Part model, mm, in its own coordinate system. A direction names the side the tool comes from. Give positions to 0.01 mm unless a question says otherwise; leave off trailing zeros. Write each loop counter-clockwise with the first axis right and the second up, starting at its lowest first coordinate (ties: lowest second). Pieces come first, ordered by that corner, then holes.
```python
from build123d import *

# Parameters (mm, degrees)
SKETCH1_W             = 3
SKETCH1_H             = 35
BOSS_EXTRUDE1_DEPTH   = 22
BOSS_EXTRUDE1_2_DEPTH = 22
SKETCH2_R             = 1.3
CUT_EXTRUDE1_DEPTH    = 45.891535951
SKETCH4_W             = 3
SKETCH4_H             = 35
BOSS_EXTRUDE3_DEPTH   = 8
BOSS_EXTRUDE4_DEPTH   = 3
SKETCH7_R             = 13.5
BOSS_EXTRUDE5_DEPTH   = 5
SKETCH8_R             = 11.75
CUT_EXTRUDE2_DEPTH    = 3
SKETCH9_R             = 2.5
CUT_EXTRUDE3_DEPTH    = 1.5
CUT_EXTRUDE4_START    = -1.5
SKETCH10_R            = 2.5
CUT_EXTRUDE4_DEPTH    = 1.5
SKETCH11_W            = 35
SKETCH11_H            = 3
BOSS_EXTRUDE6_DEPTH   = 17.5
SKETCH13_W            = 35
SKETCH13_H            = 3
BOSS_EXTRUDE7_DEPTH   = 40
SKETCH14_W            = 42
SKETCH14_H            = 27
BOSS_EXTRUDE8_DEPTH   = 3
SKETCH15_R            = 1.7
CUT_EXTRUDE5_DEPTH    = 40
FILLET1_R             = 10
FILLET2_R             = 5
FILLET3_R             = 3


with BuildPart() as part:
    # Sketch1 → Boss-Extrude1 (new body)
    with BuildSketch(Plane(origin=(0, 0, 0), x_dir=(1, 0, 0), z_dir=(0, 1, 0))):
        with Locations((-16, 0)):
            Rectangle(SKETCH1_W, SKETCH1_H)
    extrude(amount=BOSS_EXTRUDE1_DEPTH)


with BuildPart() as body_2:
    # Sketch1 → Boss-Extrude1 2 (new body)
    with BuildSketch(Plane(origin=(0, 0, 0), x_dir=(1, 0, 0), z_dir=(0, 1, 0))):
        with Locations((16, 0)):
            Rectangle(SKETCH1_W, SKETCH1_H)
    extrude(amount=BOSS_EXTRUDE1_2_DEPTH)


with BuildPart() as cut_extrude1_tool:
    # Sketch2 → Cut-Extrude1 (new, through all)
    with BuildSketch(Plane.ZY.offset(17.5)):
        with Locations((-12.5, 17)):
            Circle(SKETCH2_R)
        with Locations((11.5, 17)):
            Circle(SKETCH2_R)
        with Locations((11.5, 5)):
            Circle(SKETCH2_R)
        with Locations((-12.5, 5)):
            Circle(SKETCH2_R)
    extrude(amount=-CUT_EXTRUDE1_DEPTH)


with BuildPart() as part_1:
    add(part.part)

    # Cut-Extrude1: cut by cut_extrude1_tool
    add(cut_extrude1_tool.part, mode=Mode.SUBTRACT)



with BuildPart() as body_2_1:
    add(body_2.part)

    # Cut-Extrude1: cut by cut_extrude1_tool
    add(cut_extrude1_tool.part, mode=Mode.SUBTRACT)


with BuildPart() as part_2:
    add(part_1.part)

    add(body_2_1.part)  # Boss-Extrude3 merges body 2
    # Sketch4 → Boss-Extrude3 (add)
    with BuildSketch(Plane.XZ):
        with Locations((-16, 0)):
            Rectangle(SKETCH4_W, SKETCH4_H)
        with Locations((16, 0)):
            Rectangle(SKETCH4_W, SKETCH4_H)
    extrude(amount=BOSS_EXTRUDE3_DEPTH)

    # Sketch5 → Boss-Extrude4 (add)
    with BuildSketch(Plane.XZ.offset(8)):
        Polygon((-17.5, 17.5), (17.5, 17.5), (17.5, -17.5), (7.5, -17.5), (7.5, 0), (-7.5, 0), (-7.5, -17.5), (-17.5, -17.5), align=None)
    extrude(amount=BOSS_EXTRUDE4_DEPTH)

    # Sketch7 → Boss-Extrude5 (add)
    with BuildSketch(Plane.XZ.offset(11)):
        with Locations(Location((0, 16.5, 0), (0, 0, 175.751977333))):
            Circle(SKETCH7_R)
    extrude(amount=BOSS_EXTRUDE5_DEPTH)

    # Sketch8 → Cut-Extrude2 (cut)
    with BuildSketch(Plane(origin=(0, -16, 0), x_dir=(-1, 0, 0), z_dir=(0, -1, 0))):
        with Locations(Location((0, -16.5, 0), (0, 0, 90))):
            Circle(SKETCH8_R)
    extrude(amount=-CUT_EXTRUDE2_DEPTH, mode=Mode.SUBTRACT)

    # Sketch9 → Cut-Extrude3 (cut)
    with BuildSketch(Plane.ZY.offset(17.5)):
        with Locations((-12.5, 17)):
            Circle(SKETCH9_R)
        with Locations((11.5, 17)):
            Circle(SKETCH9_R)
        with Locations((11.5, 5)):
            Circle(SKETCH9_R)
        with Locations((-12.5, 5)):
            Circle(SKETCH9_R)
    extrude(amount=-CUT_EXTRUDE3_DEPTH, mode=Mode.SUBTRACT)

    # Sketch10 → Cut-Extrude4 (cut)
    with BuildSketch(Plane(origin=(17.5, 0, 0), x_dir=(0, 0, -1), z_dir=(1, 0, 0)).offset(CUT_EXTRUDE4_START)):
        with Locations(Location((-11.5, 17, 0), (0, 0, 180))):
            Circle(SKETCH10_R)
        with Locations(Location((12.5, 17, 0), (0, 0, 180))):
            Circle(SKETCH10_R)
        with Locations(Location((12.5, 5, 0), (0, 0, 180))):
            Circle(SKETCH10_R)
        with Locations(Location((-11.5, 5, 0), (0, 0, 180))):
            Circle(SKETCH10_R)
    extrude(amount=CUT_EXTRUDE4_DEPTH, mode=Mode.SUBTRACT)

    # Sketch11 → Boss-Extrude6 (add)
    with BuildSketch(Plane.XY.offset(17.5)):
        with Locations((0, -9.5)):
            Rectangle(SKETCH11_W, SKETCH11_H)
    extrude(amount=BOSS_EXTRUDE6_DEPTH)

    # Sketch13 → Boss-Extrude7 (add)
    with BuildSketch(Plane.XZ.offset(11)):
        with Locations((0, 33.5)):
            Rectangle(SKETCH13_W, SKETCH13_H)
    extrude(amount=BOSS_EXTRUDE7_DEPTH)

    # Sketch14 → Boss-Extrude8 (add)
    with BuildSketch(Plane.XY.offset(35)):
        with Locations((0, -37.5)):
            Rectangle(SKETCH14_W, SKETCH14_H)
    extrude(amount=-BOSS_EXTRUDE8_DEPTH)

    # Sketch15 → Cut-Extrude5 (cut)
    with BuildSketch(Plane.XY.offset(35)):
        with Locations((-16, -29)):
            Circle(SKETCH15_R)
        with Locations((16, -29)):
            Circle(SKETCH15_R)
        with Locations((16, -46)):
            Circle(SKETCH15_R)
        with Locations((-16, -46)):
            Circle(SKETCH15_R)
    extrude(amount=-CUT_EXTRUDE5_DEPTH, mode=Mode.SUBTRACT)

    # Fillet1
    # the kernel refuses this fillet: 10 mm, written as the material it adds along each edge
    with BuildSketch(Plane(origin=(17.5, -11, 32), x_dir=(0, 0, -1), z_dir=(-1, 0, 0))) as fillet1_piece_1_section:
        with BuildLine():
            CenterArc((FILLET1_R, FILLET1_R), FILLET1_R, 180, 90)
            Line((0, FILLET1_R), (0, 0))
            Line((0, 0), (FILLET1_R, 0))
        make_face()
    fillet1_piece_1 = extrude(amount=35, mode=Mode.PRIVATE)
    fillet1_piece_1 = fillet1_piece_1 - Plane(origin=(0, -11, 16.5), x_dir=(0, 0, -1), z_dir=(0, -1, 0)) * Cylinder(11.75, 110, mode=Mode.PRIVATE)
    add(fillet1_piece_1)

    # Fillet2
    # the kernel refuses this fillet: 5 mm, written as the material it adds along each edge
    with BuildSketch(Plane(origin=(14.5, -8, 17.5), x_dir=(0, 0, 1), z_dir=(1, 0, 0)), Plane(origin=(-17.5, -8, 17.5), x_dir=(0, 0, 1), z_dir=(1, 0, 0))) as fillet2_piece_1:
        with BuildLine():
            CenterArc((FILLET2_R, -FILLET2_R), FILLET2_R, 90, 90)
            Line((0, -FILLET2_R), (0, 0))
            Line((0, 0), (FILLET2_R, 0))
        make_face()
    extrude(amount=3)
    with BuildSketch(Plane(origin=(-7.5, -8, 0), x_dir=(0, 0, -1), z_dir=(0, -1, 0)), Plane(origin=(7.5, -8, 0), x_dir=(-1, 0, 0), z_dir=(0, -1, 0))) as fillet2_piece_2:
        with BuildLine():
            CenterArc((FILLET2_R, FILLET2_R), FILLET2_R, 180, 90)
            Line((0, FILLET2_R), (0, 0))
            Line((0, 0), (FILLET2_R, 0))
        make_face()
    extrude(amount=3)
    # the kernel refuses this fillet: 5 mm, written as the material it takes off along each edge
    with BuildSketch(Plane(origin=(-30, 22, 17.5), x_dir=(0, 0, -1), z_dir=(1, 0, 0)), Plane(origin=(21, -51, 47.5), x_dir=(0, 1, 0), z_dir=(0, 0, -1)), Plane(origin=(-21, -51, 47.5), x_dir=(1, 0, 0), z_dir=(0, 0, -1)), Plane(origin=(-7.5, 4.5, -17.5), x_dir=(-1, 0, 0), z_dir=(0, -1, 0)), Plane(origin=(7.5, 4.5, -17.5), x_dir=(0, 0, 1), z_dir=(0, -1, 0)), Plane(origin=(2, 22, -17.5), x_dir=(0, -1, 0), z_dir=(1, 0, 0))) as fillet2_2_piece_1:
        with BuildLine():
            CenterArc((FILLET2_R, -FILLET2_R), FILLET2_R, 90, 90)
            Line((0, -FILLET2_R), (0, 0))
            Line((0, 0), (FILLET2_R, 0))
        make_face()
    extrude(amount=28, mode=Mode.SUBTRACT)
    with BuildSketch(Plane(origin=(30, 22, 17.5), x_dir=(0, 0, -1), z_dir=(-1, 0, 0)), Plane(origin=(-2, 22, -17.5), x_dir=(0, -1, 0), z_dir=(-1, 0, 0))) as fillet2_2_piece_2:
        with BuildLine():
            CenterArc((FILLET2_R, FILLET2_R), FILLET2_R, 180, 90)
            Line((0, FILLET2_R), (0, 0))
            Line((0, 0), (FILLET2_R, 0))
        make_face()
    extrude(amount=28, mode=Mode.SUBTRACT)
    with BuildSketch(Plane(origin=(-21, -24, 46.924240018), x_dir=(0, -1, 0), z_dir=(0, 0, -1))) as fillet2_2_piece_3:
        with BuildLine():
            CenterArc((4.769696007, -5), FILLET2_R, 90, 72.542396876)
            Line((0, -3.5), (0, 0))
            Line((0, 0), (4.769696007, 0))
        make_face()
    extrude(amount=26.848480035, mode=Mode.SUBTRACT)
    with BuildSketch(Plane(origin=(21, -24, 46.924240018), x_dir=(-1, 0, 0), z_dir=(0, 0, -1))) as fillet2_2_piece_4:
        with BuildLine():
            CenterArc((5, -4.769696007), FILLET2_R, 107.457603124, 72.542396876)
            Line((0, -4.769696007), (0, 0))
            Line((0, 0), (3.5, 0))
        make_face()
    extrude(amount=26.848480035, mode=Mode.SUBTRACT)

    # Fillet3
    fillet3_edges = [part_2.edges().sort_by_distance(p)[0] for p in [
        (0, -8, 35),
    ]]
    fillet(fillet3_edges, radius=FILLET3_R)


solid = part_2.part
```
1) Saw through at A-A, the plane z = -9. Write the cut outline in (x, y), then the cut area to 3 significant figures.
Answers follow:
outline: (-17.5, -11) - (-7.5, -11) - (-7.5, -8) - (-14.5, -8) - (-14.5, 22) - (-17.5, 22) - close; (7.5, -11) - (17.5, -11) - (17.5, 22) - (14.5, 22) - (14.5, -8) - (7.5, -8) - close
area: 240 mm2
2) Saw through at D-D, the plane y = 5. Count the separate pieces of the cut face and the enclosed holes in it, then the cut area to 3 significant figures.
Answers follow:
separate pieces: 6
enclosed holes: 0
area: 164 mm2
3) 3-axis set-ups, long thin cutter, end or side, ignore diameter. For faces 4 (the face through (6.07, -9.48, -1.5)), 5 (the face through (16, 7, 17.5)), 6 (the face through (14.5, 7, -2)), 7 (the face through (16, 6, 13)): which of +Z, -Z, +X, -X, +Y, -Y reach the whole face in a straight line?
Answers follow:
face 4: -Z, +Y, -Y
face 5: +Z, +X, -X, +Y
face 6: +Z, -Z, +Y
face 7: +X
4) Saw through at B-B, the plane x = 0. Write the cut outline in (y, z), then the cut area to 3 significant figures.
Answers follow:
outline: (-51, 32) - (-21, 32) arc R10 cw to (-15, 30) - (-16, 30) - (-16, 28.25) - (-13, 28.25) - (-13, 4.75) - (-16, 4.75) - (-16, 3) - (-11, 3) - (-11, 0) - (-8, 0) - (-8, 32) arc R3 ccw to (-11, 35) - (-51, 35) - close
area: 299 mm2
5) Wall check: L1, parallel to Y at x = 15.35, z = -12.5; L2, parallel to Z at x = 16.8, y = 17; L3, parallel to Z at x = 0, y = -14.35. Give the ranges that are in metal, low to high.
Answers follow:
L1: y = -11 to 3.7, 6.3 to 15.7, 18.3 to 22
L2: z = -17.5 to -15, -10 to 9, 14 to 17.5
L3: z = 3 to 4.75, 28.25 to 35
6) Two-plate mould, pull along Z, no slides. Class faces 1 (the face through (-21, -38, 34)), 2 (the face through (-17, 5, -15)), 3 (the face through (-16, 7, 17.5)): +Z half, -Z half, draft (parallel to the pull), parting line (faces both ways), or undercut.
Answers follow:
face 1: draft
face 2: undercut
face 3: +Z half
7) Saw through at C-C, the plane z = 16.5. Write the cut outline in (x, y).
Answers follow:
outline: (-17.5, -11) - (-13.5, -11) - (-13.5, -16) - (-11.75, -16) - (-11.75, -13) - (11.75, -13) - (11.75, -16) - (13.5, -16) - (13.5, -11) - (17.5, -11) - (17.5, 20) - (14.5, 20) - (14.5, -8) - (-14.5, -8) - (-14.5, 20) - (-17.5, 20) - close
8) Pin check, flat tips, straight feed: pin 1 Ø2 at (x, z) = (-12.5, 12) entering from +Y; pin 2 Ø2 at (x, y) = (-16, -46) entering from -Z; pin 3 Ø23 at (y, z) = (-5.5, -1.5) entering from -X; pin 4 Ø2 at (y, z) = (-1, 16) entering from +X. Stop position of each tip, or through.
Answers follow:
pin 1: stops at y = -8
pin 2: passes through
pin 3: stops at x = -17.5
pin 4: stops at x = 17.5
